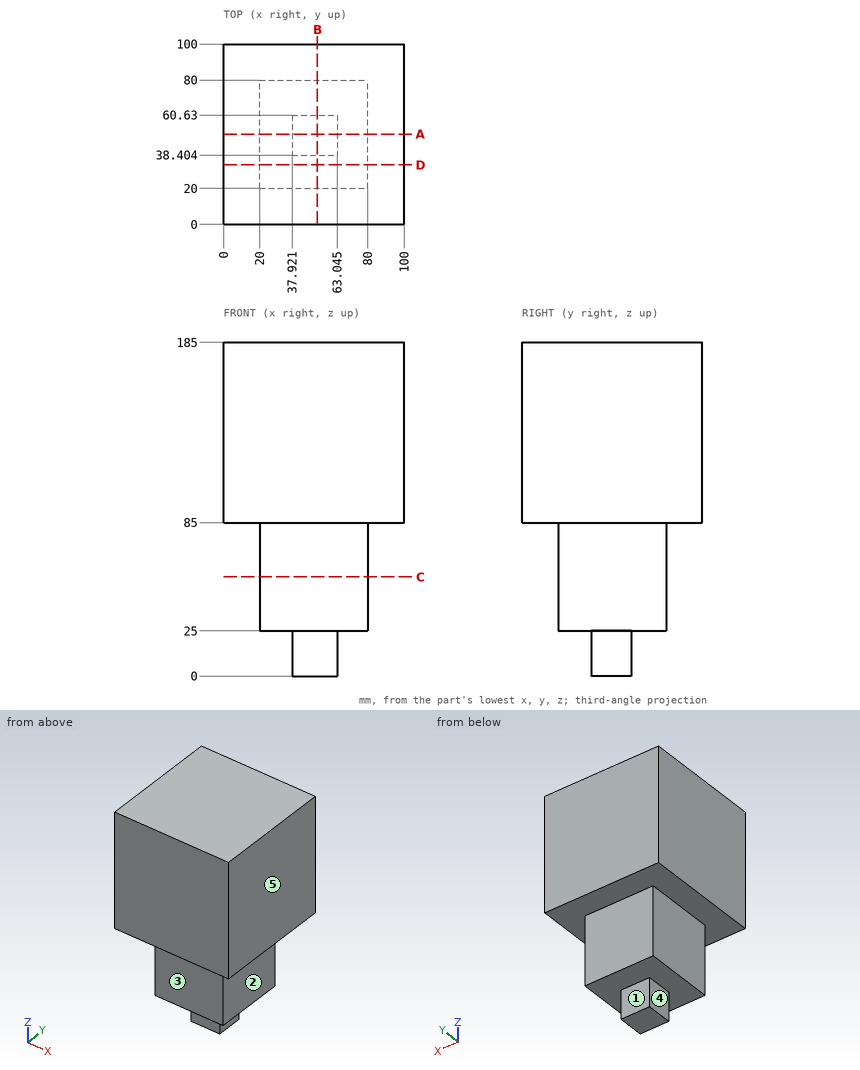
Source: three-view drawing plus pictorial views. Frame: mm from the lowest corner of the part. A direction names the side the tool comes from. Give positions to 0.01 mm unless a question says otherwise; leave off trailing zeros. Loops run counter-clockwise (first coordinate to the right, second up) from the corner with the lowest first, then second, coordinate; pieces in that order, holes last. Notation, with made-up numbers: (23.25, 89) -> (57.25, 89) arc R28 ccw to (57.25, 116) -> close; hole circle Ø6 at (52, 72.5). An arc over 180 degrees is marked (long way). Put each result on its own line as item: value. Start each with the question number.
1) Reachability of the marked faces 1, 2, 3, 4 and 5 from +Z, -Z, +X, -X, +Y, -Y: full face, straight path, thin tool, end or side. Return the list, or none.
2) Contact query for flat-ended pins moving along their axis: P1, Ø24.5, axis at y = 50.5, z = 11.5, coming from the -X side; P2, Ø1, axis at y = 68.5, z = 26, coming from the +X side; P3, Ø1.5, axis at x = 66.5, y = 20.5, coming from the -Z side. Output: stop coordinate, or through.
3) Cut plane A-A (y = 50). Return loops of the section in (x, z) (1 decimal), then the cut area to 3 significant figures.
4) Material intervals for probe 1 along Z at (x, y) = (31.5, 61); probe 2 along Y at (x, z) = (64, 30); probe 3 along Z at (x, y) = (29, 92.5), sorted ascending.
5) Cut plane D-D (y = 33). Return loops of the section in (x, z), then the cut area to 3 significant figures.
6) Cut plane C-C (z = 55). Return loops of the section in (x, y), then the cut area to 3 significant figures.
7) Cut plane B-B (x = 52). Return loops of the section in (y, z).
Results are:
1. face 1: -Z, +X, -X, +Y
1. face 2: -Z, +X, +Y, -Y
1. face 3: -Z, +X, -X, -Y
1. face 4: -Z, -X, +Y, -Y
1. face 5: +Z, -Z, +X, +Y, -Y
2. P1: stops at x = 37.92
2. P2: stops at x = 80
2. P3: stops at z = 25
3. outline: (0, 85) -> (20, 85) -> (20, 25) -> (37.9, 25) -> (37.9, 0) -> (63, 0) -> (63, 25) -> (80, 25) -> (80, 85) -> (100, 85) -> (100, 185) -> (0, 185) -> close
3. area: 14,200 mm2
4. probe 1: z = 25 to 185
4. probe 2: y = 20 to 80
4. probe 3: z = 85 to 185
5. outline: (0, 85) -> (20, 85) -> (20, 25) -> (80, 25) -> (80, 85) -> (100, 85) -> (100, 185) -> (0, 185) -> close
5. area: 13,600 mm2
6. outline: (20, 20) -> (80, 20) -> (80, 80) -> (20, 80) -> close
6. area: 3,600 mm2
7. outline: (0, 85) -> (20, 85) -> (20, 25) -> (38.4, 25) -> (38.4, 0) -> (60.63, 0) -> (60.63, 25) -> (80, 25) -> (80, 85) -> (100, 85) -> (100, 185) -> (0, 185) -> close
